```python
from build123d import *

# Parameters (mm, degrees)
SKETCH_1_R          = 5
EXTRUDE_1_DEPTH     = 100
CUT_EXTRUDE_1_DEPTH = 35


with BuildPart() as part:
    # 草图1 → 凸台-拉伸1 (new body)
    with BuildSketch(Plane(origin=(0, 0, 0), x_dir=(0, 0, -1), z_dir=(1, 0, 0))):
        Circle(SKETCH_1_R)
    extrude(amount=EXTRUDE_1_DEPTH)

    # 草图2 → 切除-拉伸1 (cut)
    with BuildSketch(Plane(origin=(100, 0, 0), x_dir=(0, 0, -1), z_dir=(1, 0, 0))):
        Polygon((0, 1), (7.225106676, 1), (7.225106676, -1), (-6.455679515, -1), (-6.455679515, 1), align=None)
    extrude(amount=-CUT_EXTRUDE_1_DEPTH, mode=Mode.SUBTRACT)

    # 镜向1: part across plane


with BuildPart() as part_1:
    add(part.part)
    add(part.part.mirror(Plane(origin=(0, 0, 0), x_dir=(0, 0, 1), z_dir=(1, 0, 0))))


solid = part_1.part
```
Can you work these out from the model? Positions are in its coordinate system, mm. A direction names the side the tool comes from. Coordinates: 2 decimals unless noted, no trailing zeros. Loops run counter-clockwise (first coordinate to the right, second up) from the corner with the lowest first, then second, coordinate; pieces in that order, holes last. Notation, with made-up numbers: (12.25, -4) - (45.25, -4) arc R17 ccw to (45.25, 27) - close; hole circle Ø2 at (68.5, 17). An arc over 180 degrees is marked (long way). Use a Markdown table: item, result.
Item 1: I want a section at C-C on y = -2.75. Please give me the cut outline in (x, z), and give its area (3 significant figures).
Numbers:
| item | result |
|---|---|
| outline | (-100, -4.18) - (100, -4.18) - (100, 4.18) - (-100, 4.18) - close |
| area | 1,670 mm2 |
Item 2: I want a section at B-B on x = -17. Please give me the cut outline in (y, z), and give its area (3 significant figures).
Numbers:
| item | result |
|---|---|
| outline | circle Ø10 at (0, 0) |
| area | 78.5 mm2 |
Item 3: If I drill on probe 1 along Z at (x, y) = (10, 1); probe 2 along X at (y, z) = (0.5, 3); probe 3 along Y at (x, z) = (-22.5, -0.25), over which ranges is the centre line in solid material (lowest first)? Write a range as from..to.
Numbers:
| item | result |
|---|---|
| probe 1 | z = -4.9..4.9 |
| probe 2 | x = -65..65 |
| probe 3 | y = -4.99..4.99 |
Item 4: For faces 1 (the face through (-100, 3, 0)), 2 (the face through (-83, -1, 0)), 3 (the face through (83, 1, 0)), which set-ups out of +Z, -Z, +X, -X, +Y, -Y let a thin tool reach every point of the face, with its end or its side?
Numbers:
| item | result |
|---|---|
| face 1 | +Z, -Z, -X, +Y, -Y |
| face 2 | +Z, -Z, -X |
| face 3 | +Z, -Z, +X |
Item 5: We'd pull the mould along Y, two halves only. Please class faces 4 (the face through (100, -3, 0)), 5 (the face through (-83, 1, 0)): released by +Y, released by -Y, zero draft, split by the parting line, or undercut.
Numbers:
| item | result |
|---|---|
| face 4 | zero draft |
| face 5 | undercut |
Item 6: I want a section at A-A on z = 0. Please give me the cut outline in (x, y), and give its area (3 significant figures).
Numbers:
| item | result |
|---|---|
| outline | (-100, -5) - (100, -5) - (100, -1) - (65, -1) - (65, 1) - (100, 1) - (100, 5) - (-100, 5) - (-100, 1) - (-65, 1) - (-65, -1) - (-100, -1) - close |
| area | 1,860 mm2 |
Item 7: Will these pins go through, and if not, where does the flat tip stop? pin 1 (1.5 mm diameter, centred on x = -17.5, z = -3, fed in from -Y); pin 2 (1.5 mm diameter, centred on x = 73.5, y = 1, fed in from -Z); pin 3 (2 mm diameter, centred on x = 10.5, y = 2.5, fed in from +Z).
Numbers:
| item | result |
|---|---|
| pin 1 | stops at y = -4.47 |
| pin 2 | stops at z = -4.9 |
| pin 3 | stops at z = 4.77 |
